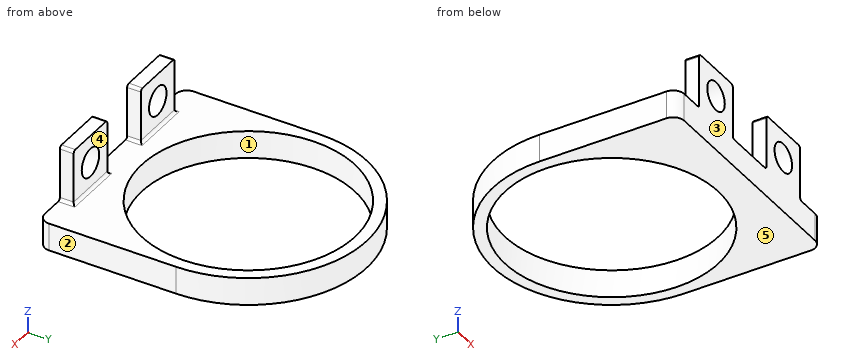
```python
from build123d import *

# Parameters (mm, degrees)
SKETCH1_R           = 24.511
BOSS_EXTRUDE1_DEPTH = 6.35
SKETCH6_W           = 12.7
SKETCH6_H           = 19.05
BOSS_EXTRUDE3_DEPTH = 3.175
SKETCH7_R           = 3.302
CUT_EXTRUDE5_DEPTH  = 65.96524836
FILLET2_R           = 0.635
FILLET3_R           = 2.54


with BuildPart() as part:
    # Sketch1 → Boss-Extrude1 (new body)
    with BuildSketch(Plane.XY):
        with BuildLine():
            Line((-27.2415, 0), (-27.2415, -31.75))
            Line((-27.2415, -31.75), (27.2415, -31.75))
            Line((27.2415, -31.75), (27.2415, 0))
            ThreePointArc((27.2415, 0), (0, 27.2415), (-27.2415, 0))
        make_face()
        Circle(SKETCH1_R, mode=Mode.SUBTRACT)
    extrude(amount=BOSS_EXTRUDE1_DEPTH)

    # Sketch6 → Boss-Extrude3 (add)
    with BuildSketch(Plane(origin=(0, -31.75, 0), x_dir=(-1, 0, 0), z_dir=(0, -1, 0))):
        with Locations((12.7, -9.525)):
            Rectangle(SKETCH6_W, SKETCH6_H)
        with Locations((-12.7, -9.525)):
            Rectangle(SKETCH6_W, SKETCH6_H)
    extrude(amount=-BOSS_EXTRUDE3_DEPTH)

    # Sketch7 → Cut-Extrude5 (cut, through all)
    with BuildSketch(Plane(origin=(0, -28.575, 0), x_dir=(1, 0, 0), z_dir=(0, 1, 0))):
        with Locations(Location((-12.7, -12.7, 0), (0, 0, 270))):
            Circle(SKETCH7_R)
        with Locations(Location((12.7, -12.7, 0), (0, 0, 270))):
            Circle(SKETCH7_R)
    extrude(amount=-CUT_EXTRUDE5_DEPTH, mode=Mode.SUBTRACT)

    # Fillet2
    fillet2_edges = [part.edges().sort_by_distance(p)[0] for p in [
        (-6.35, -30.1625, 6.35),
        (-6.35, -30.1625, 19.05),
        (-19.05, -30.1625, 6.35),
        (-19.05, -30.1625, 19.05),
        (-12.7, -28.575, 6.35),
        (12.7, -28.575, 6.35),
        (19.05, -30.1625, 6.35),
        (19.05, -30.1625, 19.05),
        (6.35, -30.1625, 6.35),
        (6.35, -30.1625, 19.05),
    ]]
    fillet(fillet2_edges, radius=FILLET2_R)

    # Fillet3
    fillet3_edges = [part.edges().sort_by_distance(p)[0] for p in [
        (27.2415, -31.75, 3.175),
        (-27.2415, -31.75, 3.175),
    ]]
    fillet(fillet3_edges, radius=FILLET3_R)


solid = part.part
```
Input: part model. Units: mm. Frame: model coordinates. Face numbers are marked on the shaded views. A direction names the side the tool comes from. Coordinates: 2 decimals unless noted, no trailing zeros. Loops run counter-clockwise (first coordinate to the right, second up) from the corner with the lowest first, then second, coordinate; pieces in that order, holes last. Notation, with made-up numbers: (45, -30.75) -> (101, -30.75) arc R31 cw to (101, -5.75) -> close; hole circle Ø4 at (-5, -7). An arc over 180 degrees is marked (long way). Use a Markdown table: item, result.
1) Cut plane D-D (y = 23). Return the cut outline in (x, z), then the cut area to 3 significant figures.
Results found:
| item | result |
|---|---|
| outline | (-14.6, 0) -> (-8.47, 0) -> (-8.47, 6.35) -> (-14.6, 6.35) -> close; (8.47, 0) -> (14.6, 0) -> (14.6, 6.35) -> (8.47, 6.35) -> close |
| area | 77.8 mm2 |
2) Cut plane B-B (x = -12.7). Return the cut outline in (y, z) (3 decimals).
Results found:
| item | result |
|---|---|
| outline | (-31.75, 0) -> (-20.964, 0) -> (-20.964, 6.35) -> (-27.94, 6.35) arc R0.635 cw to (-28.575, 6.985) -> (-28.575, 9.398) -> (-31.75, 9.398) -> close; (-31.75, 16.002) -> (-28.575, 16.002) -> (-28.575, 19.05) -> (-31.75, 19.05) -> close; (20.964, 0) -> (24.1, 0) -> (24.1, 6.35) -> (20.964, 6.35) -> close |
3) Cut plane C-C (y = -3). Return the cut outline in (x, z), then the cut area to 3 significant figures.
Results found:
| item | result |
|---|---|
| outline | (-27.24, 0) -> (-24.33, 0) -> (-24.33, 6.35) -> (-27.24, 6.35) -> close; (24.33, 0) -> (27.24, 0) -> (27.24, 6.35) -> (24.33, 6.35) -> close |
| area | 37.0 mm2 |
4) Cut plane A-A (z = 12.7). Return the cut outline in (x, y) (3 decimals), then the cut area to 3 significant figures.
Results found:
| item | result |
|---|---|
| outline | (-19.05, -31.75) -> (-16.002, -31.75) -> (-16.002, -28.575) -> (-19.05, -28.575) -> close; (-9.398, -31.75) -> (-6.35, -31.75) -> (-6.35, -28.575) -> (-9.398, -28.575) -> close; (6.35, -31.75) -> (9.398, -31.75) -> (9.398, -28.575) -> (6.35, -28.575) -> close; (16.002, -31.75) -> (19.05, -31.75) -> (19.05, -28.575) -> (16.002, -28.575) -> close |
| area | 38.7 mm2 |
5) Material intervals for line 1 along X through (y, z) = (-30.4, 12.7); line 2 along Z through (x, y) = (14.5, -26.5); line 3 along Y through (x, z) = (14, 7.75) (3 decimals), sorted ascending. Write a range as from..to.
Results found:
| item | result |
|---|---|
| line 1 | x = -19.05..-16, -9.4..-6.35, 6.35..9.4, 16..19.05 |
| line 2 | z = 0..6.35 |
| line 3 | y = -31.75..-28.575 |
6) Access query for the marked faces 4 and 5. Directions: +Z, -Z, +X, -X, +Y, -Y. A direction counts if a zero-diameter tool reaches every point of the face in a straight line with its end or side. Return the directions, or none.
Results found:
| item | result |
|---|---|
| face 4 | +Z, +X, -X, +Y |
| face 5 | -Z, +X, -X, +Y, -Y |
7) Pull-direction query (X, two-part tool) for the marked faces 1, 2 and 3; classes: released by +X, released by -X, zero draft, split by the parting line, or undercut.
Results found:
| item | result |
|---|---|
| face 1 | undercut |
| face 2 | released by +X |
| face 3 | zero draft |
8) Contact query for flat-ended pins moving along their axis: pin 1 (3.5 mm diameter, centred on y = -29.5, z = 10, fed in from -X); pin 2 (2.5 mm diameter, centred on y = -31, z = 11.5, fed in from +X); pin 3 (8 mm diameter, centred on y = 12, z = 8.5, fed in from +X). Output: stop coordinate, or through.
Results found:
| item | result |
|---|---|
| pin 1 | stops at x = -19.05 |
| pin 2 | stops at x = 19.05 |
| pin 3 | stops at x = 25.84 |
